from build123d import *

# Parameters (mm, degrees)
SKETCH_2_W          = 26.5
SKETCH_2_H          = 14.5
EXTRUDE_1_DEPTH     = 52
SKETCH_6_W          = 22.5
SKETCH_6_H          = 10.5
CUT_EXTRUDE_1_DEPTH = 49
SKETCH_7_W          = 26.5
SKETCH_7_H          = 9.5
EXTRUDE_2_DEPTH     = 24.8
FILLET_1_R          = 5
FILLET_2_R          = 1
FILLET_4_R          = 1
FILLET_5_R          = 1
FILLET_6_R          = 1
SKETCH_8_W          = 7
SKETCH_8_H          = 9.5
CUT_EXTRUDE_2_DEPTH = 20


with BuildPart() as part:
    # ｽｹｯﾁ2 → ﾎﾞｽ - 押し出し1 (new body)
    with BuildSketch(Plane.XY):
        with Locations((13.25, 7.25)):
            Rectangle(SKETCH_2_W, SKETCH_2_H)
    extrude(amount=EXTRUDE_1_DEPTH)

    # ｽｹｯﾁ6 → ｶｯﾄ - 押し出し1 (cut)
    with BuildSketch(Plane.XY.offset(52)):
        with Locations((13.25, 7.25)):
            Rectangle(SKETCH_6_W, SKETCH_6_H)
    extrude(amount=-CUT_EXTRUDE_1_DEPTH, mode=Mode.SUBTRACT)

    # ｽｹｯﾁ7 → ﾎﾞｽ - 押し出し2 (add)
    with BuildSketch(Plane.XZ):
        with Locations((13.25, 4.75)):
            Rectangle(SKETCH_7_W, SKETCH_7_H)
    extrude(amount=EXTRUDE_2_DEPTH)

    # ﾌｨﾚｯﾄ1
    fillet_1_edges = [part.edges().sort_by_distance(p)[0] for p in [
        (13.25, 0, 9.5),
    ]]
    fillet(fillet_1_edges, radius=FILLET_1_R)

    # ﾌｨﾚｯﾄ2
    fillet_2_edges = [part.edges().sort_by_distance(p)[0] for p in [
        (26.5, 14.5, 26),
    ]]
    fillet(fillet_2_edges, radius=FILLET_2_R)

    # ﾌｨﾚｯﾄ4
    fillet_4_edges = [part.edges().sort_by_distance(p)[0] for p in [
        (26.5, -14.9, 9.5),
        (26.5, -24.8, 4.75),
        (26.5, -1.464466094, 10.964466094),
        (12.75, 14.5, 0),
        (26.207106781, 14.207106781, 0),
        (26.5, -5.65, 0),
        (26.5, 0, 33.25),
    ]]
    fillet(fillet_4_edges, radius=FILLET_4_R)

    # ﾌｨﾚｯﾄ5
    # the kernel refuses this fillet: 1 mm, written as the material it takes off along each edge
    with BuildSketch(Plane(origin=(25.5, -23.8, 8.5), x_dir=(0, -1, 0), z_dir=(0, 0, 1))) as fillet_5_piece_1_section:
        Polygon((0, 0), (FILLET_5_R, 0), (FILLET_5_R, FILLET_5_R), (0, FILLET_5_R), align=None)
    fillet_5_piece_1 = extrude(amount=FILLET_5_R, mode=Mode.PRIVATE)
    fillet_5_piece_1 = fillet_5_piece_1 - Plane(origin=(25.5, -23.8, 8.5), x_dir=(-0.7071067811865475, 0.7071067811865475, 0), z_dir=(0, 0, 1)) * Sphere(FILLET_5_R, mode=Mode.PRIVATE)
    add(fillet_5_piece_1, mode=Mode.SUBTRACT)
    with BuildSketch(Plane(origin=(25.5, -23.8, 1), x_dir=(0, -1, 0), z_dir=(0, 0, -1))) as fillet_5_piece_2_section:
        Polygon((0, 0), (FILLET_5_R, 0), (FILLET_5_R, -FILLET_5_R), (0, -FILLET_5_R), align=None)
    fillet_5_piece_2 = extrude(amount=FILLET_5_R, mode=Mode.PRIVATE)
    fillet_5_piece_2 = fillet_5_piece_2 - Plane(origin=(25.5, -23.8, 1), x_dir=(-0.7071067811865475, 0.7071067811865475, 0), z_dir=(0, 0, -1)) * Sphere(FILLET_5_R, mode=Mode.PRIVATE)
    add(fillet_5_piece_2, mode=Mode.SUBTRACT)
    with BuildSketch(Plane(origin=(1, -23.8, 8.5), x_dir=(-1, 0, 0), z_dir=(0, -1, 0))) as fillet_5_piece_3_section:
        Polygon((0, 0), (FILLET_5_R, 0), (FILLET_5_R, -FILLET_5_R), (0, -FILLET_5_R), align=None)
    fillet_5_piece_3 = extrude(amount=FILLET_5_R, mode=Mode.PRIVATE)
    fillet_5_piece_3 = fillet_5_piece_3 - Plane(origin=(1, -23.8, 8.5), x_dir=(0.7071067811865475, 0, -0.7071067811865475), z_dir=(0, -1, 0)) * Sphere(FILLET_5_R, mode=Mode.PRIVATE)
    add(fillet_5_piece_3, mode=Mode.SUBTRACT)
    with BuildSketch(Plane(origin=(1, -23.8, 1), x_dir=(-1, 0, 0), z_dir=(0, 0, -1))) as fillet_5_piece_4_section:
        Polygon((0, 0), (FILLET_5_R, 0), (FILLET_5_R, -FILLET_5_R), (0, -FILLET_5_R), align=None)
    fillet_5_piece_4 = extrude(amount=FILLET_5_R, mode=Mode.PRIVATE)
    fillet_5_piece_4 = fillet_5_piece_4 - Plane(origin=(1, -23.8, 1), x_dir=(0.7071067811865475, 0.7071067811865475, 0), z_dir=(0, 0, -1)) * Sphere(FILLET_5_R, mode=Mode.PRIVATE)
    add(fillet_5_piece_4, mode=Mode.SUBTRACT)
    with BuildSketch(Plane(origin=(0, -5, 9.5), x_dir=(0, 0, -1), z_dir=(0, -1, 0))) as fillet_5_piece_5:
        with BuildLine():
            CenterArc((FILLET_5_R, FILLET_5_R), FILLET_5_R, 180, 90)
            Line((0, FILLET_5_R), (0, 0))
            Line((0, 0), (FILLET_5_R, 0))
        make_face()
    extrude(amount=18.8, mode=Mode.SUBTRACT)
    with BuildSketch(Plane(origin=(0, -24.8, 8.5), x_dir=(0, 1, 0), z_dir=(0, 0, -1))) as fillet_5_piece_6:
        with BuildLine():
            CenterArc((FILLET_5_R, FILLET_5_R), FILLET_5_R, 180, 90)
            Line((0, FILLET_5_R), (0, 0))
            Line((0, 0), (FILLET_5_R, 0))
        make_face()
    extrude(amount=7.5, mode=Mode.SUBTRACT)
    with BuildSketch(Plane(origin=(1, -24.8, 0), x_dir=(0, 1, 0), z_dir=(1, 0, 0)), Plane(origin=(25.5, -24.8, 9.5), x_dir=(0, 1, 0), z_dir=(-1, 0, 0))) as fillet_5_piece_7:
        with BuildLine():
            CenterArc((FILLET_5_R, FILLET_5_R), FILLET_5_R, 180, 90)
            Line((0, FILLET_5_R), (0, 0))
            Line((0, 0), (FILLET_5_R, 0))
        make_face()
    extrude(amount=24.5, mode=Mode.SUBTRACT)
    with BuildSketch(Plane(origin=(0, -5, 14.5), x_dir=(0, 1, 0), z_dir=(0, 0, 1))) as fillet_5_piece_8:
        with BuildLine():
            CenterArc((5 + FILLET_5_R, -FILLET_5_R), FILLET_5_R, 90, 90)
            Line((5, -FILLET_5_R), (5, 0))
            Line((5, 0), (5 + FILLET_5_R, 0))
        make_face()
    revolve(axis=Axis((0, -5, 14.5), (-1, 0, 0)), revolution_arc=90, mode=Mode.SUBTRACT)
    with BuildSketch(Plane(origin=(0, 13.5, 0), x_dir=(0, 0, 1), z_dir=(0, -1, 0))) as fillet_5_piece_9:
        with BuildLine():
            CenterArc((FILLET_5_R, -FILLET_5_R), FILLET_5_R, 90, 90)
            Line((0, -FILLET_5_R), (0, 0))
            Line((0, 0), (FILLET_5_R, 0))
        make_face()
    extrude(amount=37.3, mode=Mode.SUBTRACT)
    with BuildSketch(Plane(origin=(0, 13.5, 1), x_dir=(0, 0, -1), z_dir=(0, -1, 0))) as fillet_5_piece_10:
        with BuildLine():
            CenterArc((1 - FILLET_5_R, FILLET_5_R), FILLET_5_R, 270, 90)
            Line((1, FILLET_5_R), (1, 0))
            Line((1, 0), (1 - FILLET_5_R, 0))
        make_face()
    revolve(axis=Axis((0, 13.5, 1), (1, 0, 0)), revolution_arc=90, mode=Mode.SUBTRACT)
    with BuildSketch(Plane(origin=(0, 14.5, 1), x_dir=(1, 0, 0), z_dir=(0, 0, 1))) as fillet_5_piece_11:
        with BuildLine():
            CenterArc((FILLET_5_R, -FILLET_5_R), FILLET_5_R, 90, 90)
            Line((0, -FILLET_5_R), (0, 0))
            Line((0, 0), (FILLET_5_R, 0))
        make_face()
    extrude(amount=53.5, mode=Mode.SUBTRACT)
    with BuildSketch(Plane(origin=(0, 0, 14.5), x_dir=(1, 0, 0), z_dir=(0, 0, 1))) as fillet_5_piece_12:
        with BuildLine():
            CenterArc((FILLET_5_R, FILLET_5_R), FILLET_5_R, 180, 90)
            Line((0, FILLET_5_R), (0, 0))
            Line((0, 0), (FILLET_5_R, 0))
        make_face()
    extrude(amount=40, mode=Mode.SUBTRACT)

    # ﾌｨﾚｯﾄ6
    fillet_6_edges = [part.edges().sort_by_distance(p)[0] for p in [
        (13.25, 14.5, 52),
        (26.207106781, 14.207106781, 52),
        (26.5, 7.25, 52),
        (26.207106781, 0.292893219, 52),
        (0, 7.25, 52),
        (13.25, 0, 52),
        (0.292893219, 0.292893219, 52),
        (0.292893219, 14.207106781, 52),
    ]]
    fillet(fillet_6_edges, radius=FILLET_6_R)

    # ｽｹｯﾁ8 → ｶｯﾄ - 押し出し2 (cut)
    with BuildSketch(Plane.XZ.offset(24.8)):
        with Locations((13.25, 4.75)):
            Rectangle(SKETCH_8_W, SKETCH_8_H)
    extrude(amount=-CUT_EXTRUDE_2_DEPTH, mode=Mode.SUBTRACT)


solid = part.part
Could you check a few things on this model? Use its own coordinates, in mm. A direction names the side the tool comes from. Coordinates: 2 decimals unless noted, no trailing zeros. Loops run counter-clockwise (first coordinate to the right, second up) from the corner with the lowest first, then second, coordinate; pieces in that order, holes last.
1. Imagine slicing it at C-C (x = 10.5). Please give me the cut outline in (y, z).
2. For P1, Ø7, axis at x = 3.5, y = -13.5, coming from the +Z side; P2, Ø3.5, axis at x = 12, z = 7, coming from the -Y side; P3, Ø5, axis at y = -2, z = 26.5, coming from the -X side; P4, Ø12, axis at y = -8.5, z = 31, coming from the -X side, each with a flat end and sliding along its axis, tell me the tip position at first contact or that it passes through.
3. For faces 1 (the face through (13, -4.8, 5)), 2 (the face through (21, -14, 9.5)), 3 (the face through (13, 2, 28)), which set-ups out of +Z, -Z, +X, -X, +Y, -Y let a thin tool reach every point of the face, with its end or its side?
4. Imagine slicing it at A-A (z = 22). Please give me the cut outline in (x, y), and give its area (3 significant figures).
5. I need wall thicknesses on L1, parallel to X at y = 4.5, z = 19.5; L2, parallel to Y at x = 17.5, z = 31; L3, parallel to Y at x = 17.75, z = 8. Which ranges of each line are inside material? Lowest first, please.
6. Imagine slicing it at D-D (y = 3). Please give me the cut outline in (x, z).
7. Imagine slicing it at B-B (y = -12). Please give me the cut outline in (x, z).
8. We'd pull the mould along Y, two halves only. Please class faces 4 (the face through (2, 7, 28)), 5 (the face through (24.5, 7, 28)), 6 (the face through (5, -14, 9.5)), 7 (the face through (5, -24.8, 5)): released by +Y, released by -Y, zero draft, split by the parting line, or undercut.
Computed values:
1. outline: (-5, 9.5) - (-4.8, 9.5) - (-4.8, 0) - (13.5, 0) arc R1 ccw to (14.5, 1) - (14.5, 51) arc R1 ccw to (13.5, 52) - (12.5, 52) - (12.5, 3) - (2, 3) - (2, 52) - (1, 52) arc R1 ccw to (0, 51) - (0, 14.5) arc R5 cw to start
2. P1: stops at z = 9.5
2. P2: stops at y = -4.8
2. P3: stops at x = 0.13
2. P4: passes through
3. face 1: -Z, -Y
3. face 2: +Z, +X, -X, -Y
3. face 3: +Z
4. outline: (0, 1) arc R1 ccw to (1, 0) - (25.5, 0) arc R1 ccw to (26.5, 1) - (26.5, 13.5) arc R1 ccw to (25.5, 14.5) - (1, 14.5) arc R1 ccw to (0, 13.5) - close; hole (2, 2) - (24.5, 2) - (24.5, 12.5) - (2, 12.5) - close
4. area: 147 mm2
5. L1: x = 0 to 2, 24.5 to 26.5
5. L2: y = 0 to 2, 12.5 to 14.5
5. L3: y = -24.8 to 2, 12.5 to 14.5
6. outline: (0, 1) arc R1 ccw to (1, 0) - (25.5, 0) arc R1 ccw to (26.5, 1) - (26.5, 51) arc R1 ccw to (25.5, 52) - (24.5, 52) - (24.5, 3) - (2, 3) - (2, 52) - (1, 52) arc R1 ccw to (0, 51) - close
7. outline: (0, 1) arc R1 ccw to (1, 0) - (9.75, 0) - (9.75, 9.5) - (1, 9.5) arc R1 ccw to (0, 8.5) - close; (16.75, 0) - (25.5, 0) arc R1 ccw to (26.5, 1) - (26.5, 8.5) arc R1 ccw to (25.5, 9.5) - (16.75, 9.5) - close
8. face 4: undercut
8. face 5: undercut
8. face 6: zero draft
8. face 7: released by -Y
